Autodesk Inventor part; units mm, degrees
ref_plane "YZ Plane" through (0, 0, 0) normal (1, 0, 0) x (0, 1, 0)
ref_plane "XZ Plane" through (0, 0, 0) normal (0, 1, 0) x (-1, 0, 0)
ref_plane "XY Plane" through (0, 0, 0) normal (0, 0, 1) x (1, 0, 0)
sketch "Sketch2" plane through (0, 0, 0) normal (0, 1, 0) x (-1, 0, 0)
  line L0 (0, 0) -> (457.2, 0)
  line L1 (457.2, 0) -> (457.2, -914.4)
  line L2 (457.2, -914.4) -> (0, -914.4)
  line L3 (0, -914.4) -> (0, 0)
  line L4 (457.2, -457.2) -> (0, -457.2)
  dimension "d2" = 457.2
  dimension "d3" = 914.4
extrude "Extrusion2" add sketch "Sketch2" along normal blind 1828.8
sketch "Sketch3" plane through (0, 0, 0) normal (1, 0, 0) x (0, 0, -1)
  line L0 (914.4, 1828.8) -> (0, 1828.8)
  line L1 (457.2, 1828.8) -> (457.2, 0)
  line L2 (914.4, 0) -> (0, 0)
sketch "Sketch4" plane through (0, 0, 0) normal (1, 0, 0) x (0, 0, -1)
  line L0 (355.1544, 1039.5953) -> (401.9558, 1039.5953)
  line L1 (401.9558, 1039.5953) -> (401.9558, 861.75)
  line L2 (401.9558, 861.75) -> (355.1544, 861.75)
  line L3 (355.1544, 861.75) -> (355.1544, 1039.5953)
  line L4 (518.9593, 861.75) -> (565.7607, 861.75)
  line L5 (565.7607, 861.75) -> (565.7607, 1039.5953)
  line L6 (565.7607, 1039.5953) -> (518.9593, 1039.5953)
  line L7 (518.9593, 1039.5953) -> (518.9593, 861.75)
  point P0 (0, 0)
extrude "Extrusion3" add sketch "Sketch4" along normal blind 50.8
sketch "Sketch5" plane through (0, 0, 0) normal (1, 0, 0) x (0, 0, -1)
  line L0 (34.1958, 1790.2512) -> (883.0565, 1790.2512)
  line L1 (883.0565, 1790.2512) -> (883.0565, 32.1843)
  line L2 (883.0565, 32.1843) -> (34.1958, 32.1843)
  line L3 (34.1958, 32.1843) -> (34.1958, 1790.2512)
  point P0 (0, 0)
properties part number "Cabinet"
The model under review builds one solid part; all positions refer to its coordinate system, in mm. A direction names the side the tool comes from. Round coordinates to 2 decimals unless told otherwise and drop trailing zeros. Order: outer loops, then holes, each group sorted by start corner. A loop starts at its lowest first (then second) coordinate and runs counter-clockwise, first axis right, second up. Notation, with made-up numbers: (55.25, 62.25) -> (86.25, 62.25) arc R4 cw to (86.25, 67.25) -> close; hole circle Ø10 at (57.25, 61.25). An arc over 180 degrees is marked (long way). Write item = value, one per line. Start each with the question number.
Item 1: Mouldability with a two-part tool opening along Z and no side actions: class faces 4 (the face through (25, 949, -565.761)), 5 (the face through (25, 952, -518.959)), 6 (the face through (25, 861.75, -379)) as released by +Z, released by -Z, zero draft, split by the parting line, or undercut.
Item 2: For faces 1 (the face through (25, 1039.595, -543)), 2 (the face through (25, 949, -355.154)), 3 (the face through (25, 952, -401.956)), list the 3-axis set-ups (+Z, -Z, +X, -X, +Y, -Y) from which the entire face can be reached by the end or side of a thin tool; tool diameter is ignored.
Item 3: Consider section A-A on x = 19.5. Write out the cut boundary in (y, z).
Item 4: For line 1 along X through (y, z) = (1489, -244), list the stretches that pass through material, from the lowest coordinate up.
Item 5: Consider section B-B on y = 916.5. Write out the cut boundary in (x, z), plus the area to 3 significant figures.
Item 6: Consider section D-D on y = 305. Write out the cut boundary in (x, z), plus the area to 3 significant figures.
Item 7: Consider section C-C on z = -794. Write out the cut boundary in (x, y).
Item 8: Clearance check with flat-ended pins moving along their axes: pin 1 Ø15 at (x, y) = (25, 925.5) entering from +Z; pin 2 Ø2 at (y, z) = (1318.5, -778) entering from +X; pin 3 Ø23.5 at (x, z) = (14.5, -541) entering from -Y. State where each tip first meets the part, or that it passes through.
Conclusion:
q1.face_4 = released by -Z
q1.face_5 = undercut
q1.face_6 = zero draft
q2.face_1 = +Z, -Z, +X, +Y
q2.face_2 = +Z, +X, +Y, -Y
q2.face_3 = +X, +Y, -Y
q3.outline = (861.75, -565.76) -> (1039.6, -565.76) -> (1039.6, -518.96) -> (861.75, -518.96) -> close; (861.75, -401.96) -> (1039.6, -401.96) -> (1039.6, -355.15) -> (861.75, -355.15) -> close
q4.line_1 = -457.2 to 0
q5.outline = (-457.2, -914.4) -> (0, -914.4) -> (0, -565.76) -> (50.8, -565.76) -> (50.8, -518.96) -> (0, -518.96) -> (0, -401.96) -> (50.8, -401.96) -> (50.8, -355.15) -> (0, -355.15) -> (0, 0) -> (-457.2, 0) -> close
q5.area = 423,000 mm2
q6.outline = (-457.2, -914.4) -> (0, -914.4) -> (0, 0) -> (-457.2, 0) -> close
q6.area = 418,000 mm2
q7.outline = (-457.2, 0) -> (0, 0) -> (0, 1828.8) -> (-457.2, 1828.8) -> close
q8.pin_1 = -355.15
q8.pin_2 = 0
q8.pin_3 = 861.75
